Could you check a few things on this model? Use its own coordinates, in mm. Give positions to 0.01 mm unless a question says otherwise; leave off trailing zeros. Write each loop counter-clockwise with the first axis right and the second up, starting at its lowest first coordinate (ties: lowest second). Pieces come first, ordered by that corner, then holes. Notation, with made-up numbers: (39, 31) - (75, 31) arc R13 cw to (75, 47) - close; hole circle Ø5 at (20.5, -38.75). An arc over 180 degrees is marked (long way). Use one line per item in the form item = value.
```python
from build123d import *

# Parameters (mm, degrees)
F0_W     = 400
F0_H     = 352
F1_DEPTH = 19
F3_DEPTH = 19.001
F5_DEPTH = 19.001
F6_W     = 166.512146
F6_H     = 21.710783
F7_DEPTH = 19.001


with BuildPart() as f1:
    # F0 (on Top) → F1 (new body)
    with BuildSketch(Plane.XY):
        with Locations((3.291806, 0)):
            Rectangle(F0_W, F0_H)
    extrude(amount=F1_DEPTH)

    # F2 (on face) → F3 (cut, through all)
    with BuildSketch(Plane.XY.offset(19)):
        with BuildLine():
            ThreePointArc((-196.708194, 129.747689), (-178.598659, 159.856691), (-147.391275, 176))
            Line((-147.391275, 176), (-196.708194, 176))
            Line((-196.708194, 176), (-196.708194, 129.747689))
        make_face()
        with BuildLine():
            Line((203.291806, 176), (148.288742, 176))
            ThreePointArc((148.288742, 176), (182.953617, 161.392464), (203.291806, 129.747689))
            Line((203.291806, 129.747689), (203.291806, 176))
        make_face()
    extrude(amount=-F3_DEPTH, mode=Mode.SUBTRACT)

    # F4 (on face) → F5 (cut, through all)
    with BuildSketch(Plane.XY.offset(19)):
        Polygon((-163.379148, -176), (-196.708194, -141.636923), (-196.708194, -176), align=None)
        Polygon((203.291806, -141.739659), (167.968541, -176), (203.291806, -176), align=None)
    extrude(amount=-F5_DEPTH, mode=Mode.SUBTRACT)

    # F6 (on face) → F7 (cut, through all)
    with BuildSketch(Plane.XY.offset(19)):
        with Locations((0, -143.512011)):
            Rectangle(F6_W, F6_H)
    extrude(amount=-F7_DEPTH, mode=Mode.SUBTRACT)


solid = f1.part
```
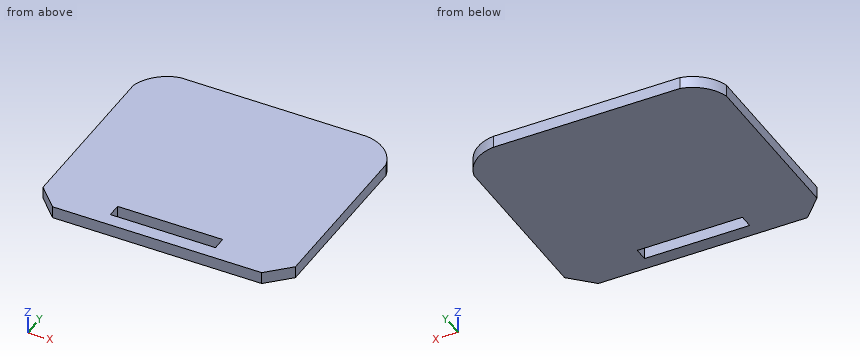
1. Imagine slicing it at C-C, the plane y = -150. List the corners of the cut face in (x, z) for me.
Response values:
outline = (-188.6, 0) - (-83.26, 0) - (-83.26, 19) - (-188.6, 19) - close; (83.26, 0) - (194.78, 0) - (194.78, 19) - (83.26, 19) - close
2. Imagine slicing it at D-D, the plane y = 151.5. List the corners of the cut face in (x, z) for me.
Response values:
outline = (-186.08, 0) - (192.43, 0) - (192.43, 19) - (-186.08, 19) - close
3. If I drill on line 1 (Y direction, x = 57.5, z = 17.75); line 2 (X direction, y = -134, z = 13); line 3 (Y direction, x = -167, z = 5.25), over which ranges is the centre line in solid material (lowest first)? Write a range as from..to.
Response values:
line_1 = -176..-154.37, -132.66..176
line_2 = -196.71..-83.26, 83.26..203.29
line_3 = -172.27..168.51
4. Imagine slicing it at B-B, the plane x = -24. List the corners of the cut face in (y, z) for me, and give its area (3 significant figures).
Response values:
outline = (-176, 0) - (-154.37, 0) - (-154.37, 19) - (-176, 19) - close; (-132.66, 0) - (176, 0) - (176, 19) - (-132.66, 19) - close
area = 6,280 mm²
5. Imagine slicing it at A-A, the plane z = 7.5. List the corners of the cut face in (x, y) for me.
Response values:
outline = (-196.71, -141.64) - (-163.38, -176) - (167.97, -176) - (203.29, -141.74) - (203.29, 129.75) arc R63.57 ccw to (148.29, 176) - (-147.39, 176) arc R64.48 ccw to (-196.71, 129.75) - close; hole (-83.26, -154.37) - (83.26, -154.37) - (83.26, -132.66) - (-83.26, -132.66) - close
6. For pin 1 (6 mm diameter, centred on y = 137.5, z = 13.5, fed in from +X), with a flat end and sliding along its axis, tell me the tip position at first contact or that it passes through.
Response values:
pin_1 = 201.77
